from build123d import *

# Parameters (mm, degrees)
SKETCH_1_R      = 1.55
SKETCH_1_W      = 10
SKETCH_1_H      = 6
SKETCH_1_R_2    = 1.5
SKETCH_1_W_2    = 15
SKETCH_1_H_2    = 6.1
SKETCH_1_W_3    = 6.1
SKETCH_1_H_3    = 10
SKETCH_1_H_4    = 15.1
EXTRUDE_1_DEPTH = 6


with BuildPart() as part:
    # Эскиз1 → Бобышка-Вытянуть1 (new body)
    with BuildSketch(Plane(origin=(0, 0, 0), x_dir=(1, 0, 0), z_dir=(0, 1, 0))):
        with BuildLine():
            Line((-168.683476523, -15.061578422), (-178.683476523, -15.061578422))
            ThreePointArc((-178.683476523, -15.061578422), (-177.790056525, -17.581332515), (-175.508896177, -18.97548726))
            Line((-175.508896177, -18.97548726), (-127.683476523, -29.061578422))
            Line((-127.683476523, -29.061578422), (62.316523477, -29.061578422))
            Line((62.316523477, -29.061578422), (110.14194313, -18.97548726))
            ThreePointArc((110.14194313, -18.97548726), (112.423103478, -17.581332515), (113.316523477, -15.061578422))
            Line((113.316523477, -15.061578422), (113.316523477, 50.938421578))
            Line((113.316523477, 50.938421578), (66.316523477, 50.938421578))
            ThreePointArc((66.316523477, 50.938421578), (63.488096352, 49.766848703), (62.316523477, 46.938421578))
            Line((62.316523477, 46.938421578), (62.316523477, 16.938421578))
            ThreePointArc((62.316523477, 16.938421578), (57.044445538, 4.210499517), (44.316523477, -1.061578422))
            Line((44.316523477, -1.061578422), (-174.683476523, -1.061578422))
            ThreePointArc((-174.683476523, -1.061578422), (-177.511903648, -2.233151297), (-178.683476523, -5.061578422))
            Line((-178.683476523, -5.061578422), (-178.683476523, -9.061578422))
            Line((-178.683476523, -9.061578422), (-168.683476523, -9.061578422))
            Line((-168.683476523, -9.061578422), (-168.683476523, -15.061578422))
        make_face()
        with Locations((-136.683476523, -12.061578422)):
            Circle(SKETCH_1_R, mode=Mode.SUBTRACT)
        with Locations((-119.683476523, -12.061578422)):
            Rectangle(SKETCH_1_W, SKETCH_1_H, mode=Mode.SUBTRACT)
        with Locations((-68.683476523, -12.061578422)):
            Circle(SKETCH_1_R, mode=Mode.SUBTRACT)
        with Locations((-38.683476523, -12.061578422)):
            Rectangle(SKETCH_1_W, SKETCH_1_H, mode=Mode.SUBTRACT)
        with Locations((-8.683476523, -12.061578422)):
            Circle(SKETCH_1_R, mode=Mode.SUBTRACT)
        with Locations((42.316523477, -12.061578422)):
            Rectangle(SKETCH_1_W, SKETCH_1_H, mode=Mode.SUBTRACT)
        with Locations((59.316523477, -12.061578422)):
            Circle(SKETCH_1_R_2, mode=Mode.SUBTRACT)
        with Locations((94.316523477, -12.061578422)):
            Rectangle(SKETCH_1_W_2, SKETCH_1_H_2, mode=Mode.SUBTRACT)
        with Locations((74.316523477, -3.061578422)):
            Circle(SKETCH_1_R_2, mode=Mode.SUBTRACT)
        with Locations((108.266523477, 7.938421578)):
            Rectangle(SKETCH_1_W_3, SKETCH_1_H_3, mode=Mode.SUBTRACT)
        with Locations((74.266523477, 16.938421578)):
            Rectangle(SKETCH_1_W_3, SKETCH_1_H_4, mode=Mode.SUBTRACT)
        with Locations((91.316523477, 16.938421578)):
            Rectangle(SKETCH_1_W, SKETCH_1_H_2, mode=Mode.SUBTRACT)
        with Locations((108.316523477, 16.938421578)):
            Circle(SKETCH_1_R_2, mode=Mode.SUBTRACT)
        with Locations((108.266523477, 25.938421578)):
            Rectangle(SKETCH_1_W_3, SKETCH_1_H_3, mode=Mode.SUBTRACT)
        with Locations((74.316523477, 36.938421578)):
            Circle(SKETCH_1_R_2, mode=Mode.SUBTRACT)
        with Locations((94.316523477, 45.938421578)):
            Rectangle(SKETCH_1_W_2, SKETCH_1_H_2, mode=Mode.SUBTRACT)
    extrude(amount=EXTRUDE_1_DEPTH)


solid = part.part
Here's how the part is built. I have some questions about the finished solid (model axes, mm). A direction names the side the tool comes from. Round coordinates to 2 decimals unless told otherwise and drop trailing zeros. Loops run counter-clockwise (first coordinate to the right, second up) from the corner with the lowest first, then second, coordinate; pieces in that order, holes last.
1. If I drill on line 1 along Z through (x, y) = (-36.5, 5.55); line 2 along X through (y, z) = (5.25, -19); line 3 along X through (y, z) = (2.7, -44.5), over which ranges is the centre line in solid material (lowest first)?
Answer list:
line 1: z = 1.06 to 9.06, 15.06 to 29.06
line 2: x = 62.32 to 71.22, 77.32 to 86.32, 96.32 to 113.32
line 3: x = 62.32 to 86.82, 101.82 to 113.32
2. If we section it at C-C on x = -155: Write out the boundary of the cut face in (y, z), plus the area to 3 significant figures.
Answer list:
outline: (0, 1.06) - (6, 1.06) - (6, 23.3) - (0, 23.3) - close
area: 133 mm2
3. For P1, Ø1.8, axis at y = 3.5, z = 12.5, coming from the -X side; P2, Ø3, axis at x = -121, y = 2, coming from the -Z side; P3, Ø1.8, axis at x = 94, y = 4.5, coming from the +Z side, each with a flat end and sliding along its axis, tell me the tip position at first contact or that it passes through.
Answer list:
P1: stops at x = -168.68
P2: stops at z = 1.06
P3: stops at z = 22.57
4. Which directions (+Z, -Z, +X, -X, +Y, -Y) give clear straight access to the entire face, cutting with the end or side of a thin tool? Please do faces 4 (the face through (86.317, 3, -17)), 5 (the face through (-64, 3, 1.062)), 6 (the face through (-34, 3, 29.062)).
Answer list:
face 4: +Y, -Y
face 5: -Z, -X, +Y, -Y
face 6: +Z, +X, -X, +Y, -Y
5. If we section it at A-A on x = -85: Write out the boundary of the cut face in (y, z).
Answer list:
outline: (0, 1.06) - (6, 1.06) - (6, 29.06) - (0, 29.06) - close
6. If we section it at B-B on y = 3.05: Count the separate pieces of the cut face and the enclosed holes in it, plus the area to 3 significant figures.
Answer list:
separate pieces: 1
enclosed holes: 16
area: 9,590 mm2
7. We'd pull the mould along X, two halves only. Please class faces 1 (the face through (-39, 3, 9.062)), 2 (the face through (86.817, 3, -46)), 3 (the face through (-2, 0, 6)): +X half, -X half, draft (parallel to the pull), parting line (faces both ways), or undercut.
Answer list:
face 1: undercut
face 2: undercut
face 3: draft
